For this review, use the dimensioned drawing (mm, ordinates from the lowest corner) and the shaded views. A direction names the side the tool comes from. Coordinates: 2 decimals unless noted, no trailing zeros. Order: outer loops, then holes, each group sorted by start corner. A loop starts at its lowest first (then second) coordinate and runs counter-clockwise, first axis right, second up. Notation, with made-up numbers: (46, -28) -> (67, -28) arc R27 ccw to (67, -5) -> close; hole circle Ø1 at (25.5, -37). An arc over 180 degrees is marked (long way). Return JSON: item names as keys, results as strings. Group by question number.
Item 1: Take a section at C-C (z = 87.5). Write out the cut boundary in (x, y).
Item 2: For line 1 along Z through (x, y) = (15.5, 32); line 2 along Y through (x, z) = (14, 41); line 3 along X through (y, z) = (21.5, 4), list the stretches that pass through material, from the lowest coordinate up.
Item 3: Machinability: for the marked faces 1 and 2, which of the approach directions +Z, -Z, +X, -X, +Y, -Y give a long, thin tool a straight path to every point of the face, cutting with its end or side? Answer none if there is none.
Item 4: Take a section at A-A (x = 20). Write out the cut boundary in (y, z).
Item 5: Insertion check: pin 1 (3 mm diameter, centred on x = 25.5, z = 36.5, fed in from -Y); pin 2 (8 mm diameter, centred on x = 12, y = 25, fed in from +Z); pin 3 (4 mm diameter, centred on x = 24, z = 27, fed in from -Y); pin 4 (2 mm diameter, centred on y = 13.5, z = 71.5, fed in from +X). Each pin has a flat end and moves straight along its axis. Give the tip position at first contact, or say it passes through.
Item 6: Take a section at B-B (z = 16.5). Write out the cut boundary in (x, y).
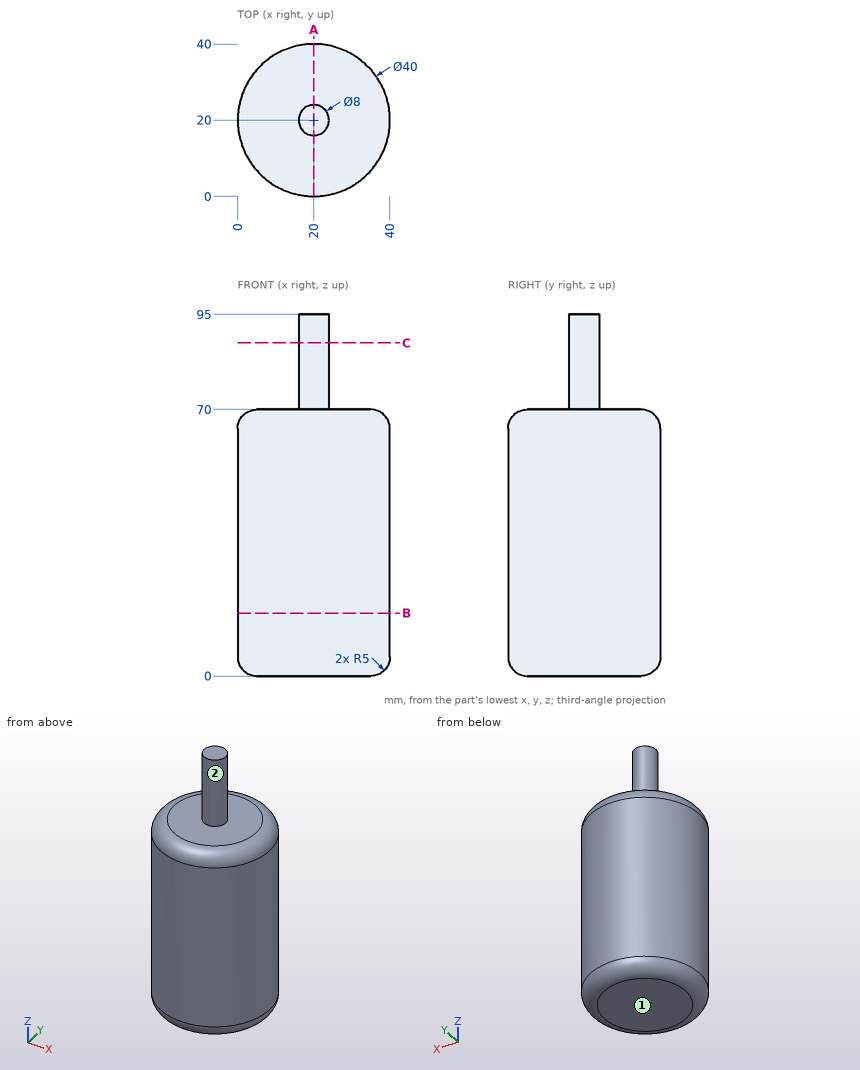
Findings below:
{
 "1": {"outline": "circle Ø8 at (20, 20)"},
 "2": {"line 1": "z = 0 to 70", "line 2": "y = 0.92 to 39.08", "line 3": "x = 0.16 to 39.84"},
 "3": {"face 1": "-Z, +X, -X, +Y, -Y", "face 2": "+Z"},
 "4": {"outline": "(0, 5) arc R5 ccw to (5, 0) -> (35, 0) arc R5 ccw to (40, 5) -> (40, 65) arc R5 ccw to (35, 70) -> (24, 70) -> (24, 95) -> (16, 95) -> (16, 70) -> (5, 70) arc R5 ccw to (0, 65) -> close"},
 "5": {"pin 1": "stops at y = 0.4", "pin 2": "stops at z = 70", "pin 3": "stops at y = 0.1", "pin 4": "passes through"},
 "6": {"outline": "circle Ø40 at (20, 20)"}
}
